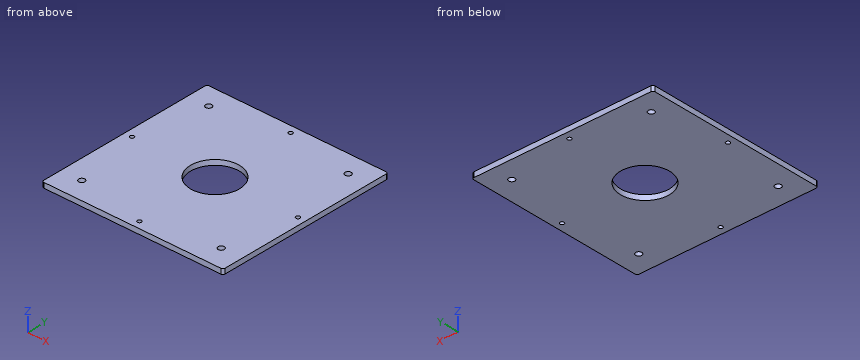
Autodesk Inventor part; units mm, degrees
ref_plane "YZ Plane" through (0, 0, 0) normal (1, 0, 0) x (0, 1, 0)
ref_plane "XZ Plane" through (0, 0, 0) normal (0, 1, 0) x (-1, 0, 0)
ref_plane "XY Plane" through (0, 0, 0) normal (0, 0, 1) x (1, 0, 0)
sketch "Sketch1" plane through (0, 0, 0) normal (0, 0, 1) x (1, 0, 0)
  line L0 (-89, 89) -> (89, 89)
  line L1 (89, 89) -> (89, -89)
  line L2 (89, -89) -> (-89, -89)
  line L3 (-89, -89) -> (-89, 89)
  circle A0 centre (0, 0) radius 24
  dimension "d33" = 178
  dimension "d34" = 89
  dimension "d35" = 89
  dimension "d65" = 48
extrude "Extrusion1" add sketch "Sketch1" along normal blind 5
sketch "Sketch2" plane through (0, 0, 5) normal (0, 0, 1) x (1, 0, 0)
  circle A0 centre (-81.5, 0) radius 2
  circle A1 centre (81.5, 0) radius 2
  line L0 (-78.5, 36.125) -> (-78.5, 56.125)
  line L1 (78.5, 56.125) -> (78.5, 36.125)
  circle A2 centre (0, 81.5) radius 2
  circle A3 centre (0, -81.5) radius 2
  line L2 (36.125, 78.5) -> (56.125, 78.5)
  line L3 (56.125, -78.5) -> (36.125, -78.5)
  line L4 (-89, 89) -> (-89, -89)
  line L5 (89, 89) -> (-89, 89)
  line L6 (89, -89) -> (89, 89)
  line L7 (-89, -89) -> (89, -89)
  point P0 (0, 0)
  point P1 (-78.5, -56.125)
  point P2 (78.5, -56.125)
  point P3 (-56.125, 78.5)
  point P4 (-56.125, -78.5)
  dimension "d18" = 4
  dimension "d37" = 7.5
  dimension "d38" = 7.5
  dimension "d39" = 7.5
  dimension "d40" = 7.5
hole "Hole1" at (-81.5, 0, 5) at (0, 81.5, 5) at (81.5, 0, 5) at (0, -81.5, 5) direction (0, 0, -1) diameter 4 end through all
fillet "Fillet1" radius 2 4 edges at (-89, -89, 2.5) (-89, 89, 2.5) (89, -89, 2.5) (89, 89, 2.5)
sketch "Sketch3" plane through (0, 0, 5) normal (0, 0, 1) x (1, 0, 0)
  line L0 (68.475, -68.475) -> (-68.475, -68.475)
  line L1 (-68.475, -68.475) -> (-68.475, 68.475)
  line L2 (-68.475, 68.475) -> (68.475, 68.475)
  line L3 (68.475, 68.475) -> (68.475, -68.475)
  line L4 (68.475, -68.475) -> (-68.475, 68.475) construction
  line L5 (-68.475, -68.475) -> (68.475, 68.475) construction
  circle A0 centre (-68.475, 68.475) radius 4.875
  point P0 (0, 0)
  dimension "d31" = 136.95
  dimension "d32" = 9.75
hole "Hole2" at (-68.475, 68.475, 5) at (68.475, 68.475, 5) at (68.475, -68.475, 5) at (-68.475, -68.475, 5) direction (0, 0, -1) diameter 6 end through all
equation "\"d38\" = d37"
equation "\"d39\" = d37"
equation "\"d40\" = d37"
equation "\"d21\" = d18"
equation "\"d6\" = 0.5 * d3"
equation "\"d7\" = 0.5 * d2"
properties part number "WaagePlexiOben3" material "PET Plastic"
Design review of the part built by this model. Coordinates are the model's own, in mm. Coordinates: 2 decimals unless noted, no trailing zeros. Loops run counter-clockwise (first coordinate to the right, second up) from the corner with the lowest first, then second, coordinate; pieces in that order, holes last. Notation, with made-up numbers: (14, 26.5) -> (51, 26.5) arc R14 cw to (51, 36.5) -> close; hole circle Ø5 at (-7, 27.25). An arc over 180 degrees is marked (long way). Use a Markdown table: item, result. Add a question column.
Item 1: Wall thickness on L1, parallel to Y at x = 0, z = 2.4; L2, parallel to Y at x = -1.5, z = 0.9; L3, parallel to X at y = 81.5, z = 3.5: over which ranges is each line inside the solid? List them lowest first. Write a range as from..to.
Item 2: We need section A-A, the plane x = -9. Write out the cut boundary in (y, z).
Item 3: We need section B-B, the plane y = -4.5. Write out the cut boundary in (x, z), and give its area (3 significant figures).
Item 4: We need section C-C, the plane z = 3.85. Count the separate pieces of the cut face and the enclosed holes in it, and give its area (3 significant figures).
Item 5: Clearance check with a flat-ended pin moving along its axis: P1, Ø5, axis at x = -68.475, y = -68.475, coming from the +Z side. State where the tip first meets the part, or that it passes through.
Numbers:
| question | item | result |
|---|---|---|
| 1 | L1 | y = -89..-83.5, -79.5..-24, 24..79.5, 83.5..89 |
| 1 | L2 | y = -89..-82.82, -80.18..-23.95, 23.95..80.18, 82.82..89 |
| 1 | L3 | x = -89..-2, 2..89 |
| 2 | outline | (-89, 0) -> (-22.25, 0) -> (-22.25, 5) -> (-89, 5) -> close; (22.25, 0) -> (89, 0) -> (89, 5) -> (22.25, 5) -> close |
| 3 | outline | (-89, 0) -> (-23.57, 0) -> (-23.57, 5) -> (-89, 5) -> close; (23.57, 0) -> (89, 0) -> (89, 5) -> (23.57, 5) -> close |
| 3 | area | 654 mm^2 |
| 4 | separate pieces | 1 |
| 4 | enclosed holes | 9 |
| 4 | area | 29,700 mm^2 |
| 5 | P1 | passes through |
